Build history of the part. All positions in model axes, mm. A direction names the side the tool comes from. Give positions to 0.01 mm unless a question says otherwise; leave off trailing zeros. Write each loop counter-clockwise with the first axis right and the second up, starting at its lowest first coordinate (ties: lowest second). Pieces come first, ordered by that corner, then holes. Notation, with made-up numbers: (-9.5, -31) -> (44.5, -31) arc R19 ccw to (44.5, 1) -> close; hole circle Ø6 at (-4, 74.25). An arc over 180 degrees is marked (long way). Put each result on its own line as item: value. Start each with the question number.
Item 1: Two-plate mould, pull along X, no slides. Class faces 6 (the cylindrical face through (2.21, -8.26, -1.33)), 7 (the flat face through (0, 0, 1)), 8 (the cylindrical face through (6.31, 10.906, -1.331)): pulls with the +X half, pulls with the -X half, needs draft (parallel to the pull), parting line crosses it, or undercut.
Item 2: Drill centre lines: line 1 along Y through (x, z) = (0, -3.1); line 2 along Y through (x, z) = (-9, -2.3); line 3 along Y through (x, z) = (-9.5, -1.75). Where is each one in solid material? Low to high.
Item 3: Slice it at C-C, the plane y = -10. Give the number of separate pieces and of enclosed holes in the cut face, plus the area to 3 significant figures.
Item 4: Slice it at A-A, the plane x = 0. List the corners of the cut face in (y, z), plus the area to 3 significant figures.
Item 5: Tool access for faces 1 (the cylindrical face through (8.257, -2.219, -1.331)), 2 (the cylindrical face through (-8.26, -2.21, -1.33)), 3 (the cylindrical face through (-2.21, 8.26, -1.33)), 4 (the cylindrical face through (-2.219, -8.257, -1.331)), 5 (the cylindrical face through (0.54, -2.44, -3.1)): list every direction of +Z, -Z, +X, -X, +Y, -Y with a clear straight run to the whole face (end or side of a thin tool).
```python
from build123d import *

# Parameters (mm, degrees)
EXTRUDE_1_DEPTH      = 1
EXTRUDE_1_DEPTH_BACK = 3.597865908
SKETCH_2_R           = 2.5
CUT_EXTRUDE_1_DEPTH  = 1


with BuildPart() as part:
    # 草图1 → 凸台-拉伸1 (new, two sides: drawn at the far end of the back side and taken through both)
    with BuildSketch(Plane.XY.offset(-EXTRUDE_1_DEPTH_BACK)):
        with BuildLine():
            ThreePointArc((-2.640449702, -8.132067718), (-2.212902836, -8.258665815), (-1.779337339, -8.36280208))
            add(Edge.make_bspline(
                [(-0.798942675, -12.574644751), (-1.838065444, -11.330781503), (-1.08287755, -9.669464778), (-1.779337339, -8.36280208)],
                knots=[0, 0, 0, 0, 1, 1, 1, 1], degree=3))
            ThreePointArc((-0.798942675, -12.574644751), (0, -12.6), (0.798942675, -12.574644751))
            add(Edge.make_bspline(
                [(0.798942675, -12.574644751), (1.838065444, -11.330781503), (1.08287755, -9.669464778), (1.779337339, -8.36280208)],
                knots=[0, 0, 0, 0, 1, 1, 1, 1], degree=3))
            ThreePointArc((1.779337339, -8.36280208), (2.212902836, -8.258665815), (2.640449702, -8.132067718))
            add(Edge.make_bspline(
                [(5.595417723, -11.289433135), (4.073579383, -10.731777349), (3.896932922, -8.915440914), (2.640449702, -8.132067718)],
                knots=[0, 0, 0, 0, 1, 1, 1, 1], degree=3))
            ThreePointArc((5.595417723, -11.289433135), (6.3, -10.911920088), (6.979227028, -10.49049046))
            add(Edge.make_bspline(
                [(6.979227028, -10.49049046), (7.25720212, -8.893711904), (5.772531856, -7.832563364), (5.722352378, -6.352730379)],
                knots=[0, 0, 0, 0, 1, 1, 1, 1], degree=3))
            ThreePointArc((5.722352378, -6.352730379), (6.045762979, -6.045762979), (6.352730379, -5.722352378))
            add(Edge.make_bspline(
                [(10.49049046, -6.979227028), (8.893711904, -7.25720212), (7.832563364, -5.772531856), (6.352730379, -5.722352378)],
                knots=[0, 0, 0, 0, 1, 1, 1, 1], degree=3))
            ThreePointArc((10.49049046, -6.979227028), (10.911920088, -6.3), (11.289433135, -5.595417723))
            add(Edge.make_bspline(
                [(11.289433135, -5.595417723), (10.731777349, -4.073579383), (8.915440914, -3.896932922), (8.132067718, -2.640449702)],
                knots=[0, 0, 0, 0, 1, 1, 1, 1], degree=3))
            ThreePointArc((8.132067718, -2.640449702), (8.258665815, -2.212902836), (8.36280208, -1.779337339))
            add(Edge.make_bspline(
                [(12.574644751, -0.798942675), (11.330781503, -1.838065444), (9.669464778, -1.08287755), (8.36280208, -1.779337339)],
                knots=[0, 0, 0, 0, 1, 1, 1, 1], degree=3))
            ThreePointArc((12.574644751, -0.798942675), (12.6, 0), (12.574644751, 0.798942675))
            add(Edge.make_bspline(
                [(12.574644751, 0.798942675), (11.330781503, 1.838065444), (9.669464778, 1.08287755), (8.36280208, 1.779337339)],
                knots=[0, 0, 0, 0, 1, 1, 1, 1], degree=3))
            ThreePointArc((8.36280208, 1.779337339), (8.258665815, 2.212902836), (8.132067718, 2.640449702))
            add(Edge.make_bspline(
                [(11.289433135, 5.595417723), (10.731777349, 4.073579383), (8.915440914, 3.896932922), (8.132067718, 2.640449702)],
                knots=[0, 0, 0, 0, 1, 1, 1, 1], degree=3))
            ThreePointArc((11.289433135, 5.595417723), (10.911920088, 6.3), (10.49049046, 6.979227028))
            add(Edge.make_bspline(
                [(10.49049046, 6.979227028), (8.893711904, 7.25720212), (7.832563364, 5.772531856), (6.352730379, 5.722352378)],
                knots=[0, 0, 0, 0, 1, 1, 1, 1], degree=3))
            ThreePointArc((6.352730379, 5.722352378), (6.045762979, 6.045762979), (5.722352378, 6.352730379))
            add(Edge.make_bspline(
                [(6.979227028, 10.49049046), (7.25720212, 8.893711904), (5.772531856, 7.832563364), (5.722352378, 6.352730379)],
                knots=[0, 0, 0, 0, 1, 1, 1, 1], degree=3))
            ThreePointArc((6.979227028, 10.49049046), (6.3, 10.911920088), (5.595417723, 11.289433135))
            add(Edge.make_bspline(
                [(5.595417723, 11.289433135), (4.073579383, 10.731777349), (3.896932922, 8.915440914), (2.640449702, 8.132067718)],
                knots=[0, 0, 0, 0, 1, 1, 1, 1], degree=3))
            ThreePointArc((2.640449702, 8.132067718), (2.212902836, 8.258665815), (1.779337339, 8.36280208))
            add(Edge.make_bspline(
                [(0.798942675, 12.574644751), (1.838065444, 11.330781503), (1.08287755, 9.669464778), (1.779337339, 8.36280208)],
                knots=[0, 0, 0, 0, 1, 1, 1, 1], degree=3))
            ThreePointArc((0.798942675, 12.574644751), (0, 12.6), (-0.798942675, 12.574644751))
            add(Edge.make_bspline(
                [(-0.798942675, 12.574644751), (-1.838065444, 11.330781503), (-1.08287755, 9.669464778), (-1.779337339, 8.36280208)],
                knots=[0, 0, 0, 0, 1, 1, 1, 1], degree=3))
            ThreePointArc((-1.779337339, 8.36280208), (-2.212902836, 8.258665815), (-2.640449702, 8.132067718))
            add(Edge.make_bspline(
                [(-5.595417723, 11.289433135), (-4.073579383, 10.731777349), (-3.896932922, 8.915440914), (-2.640449702, 8.132067718)],
                knots=[0, 0, 0, 0, 1, 1, 1, 1], degree=3))
            ThreePointArc((-5.595417723, 11.289433135), (-6.3, 10.911920088), (-6.979227028, 10.49049046))
            add(Edge.make_bspline(
                [(-6.979227028, 10.49049046), (-7.25720212, 8.893711904), (-5.772531856, 7.832563364), (-5.722352378, 6.352730379)],
                knots=[0, 0, 0, 0, 1, 1, 1, 1], degree=3))
            ThreePointArc((-5.722352378, 6.352730379), (-6.045762979, 6.045762979), (-6.352730379, 5.722352378))
            add(Edge.make_bspline(
                [(-10.49049046, 6.979227028), (-8.893711904, 7.25720212), (-7.832563364, 5.772531856), (-6.352730379, 5.722352378)],
                knots=[0, 0, 0, 0, 1, 1, 1, 1], degree=3))
            ThreePointArc((-10.49049046, 6.979227028), (-10.911920088, 6.3), (-11.289433135, 5.595417723))
            add(Edge.make_bspline(
                [(-11.289433135, 5.595417723), (-10.731777349, 4.073579383), (-8.915440914, 3.896932922), (-8.132067718, 2.640449702)],
                knots=[0, 0, 0, 0, 1, 1, 1, 1], degree=3))
            ThreePointArc((-8.132067718, 2.640449702), (-8.258665815, 2.212902836), (-8.36280208, 1.779337339))
            add(Edge.make_bspline(
                [(-12.574644751, 0.798942675), (-11.330781503, 1.838065444), (-9.669464778, 1.08287755), (-8.36280208, 1.779337339)],
                knots=[0, 0, 0, 0, 1, 1, 1, 1], degree=3))
            ThreePointArc((-12.574644751, 0.798942675), (-12.6, 0), (-12.574644751, -0.798942675))
            add(Edge.make_bspline(
                [(-12.574644751, -0.798942675), (-11.330781503, -1.838065444), (-9.669464778, -1.08287755), (-8.36280208, -1.779337339)],
                knots=[0, 0, 0, 0, 1, 1, 1, 1], degree=3))
            ThreePointArc((-8.36280208, -1.779337339), (-8.258665815, -2.212902836), (-8.132067718, -2.640449702))
            add(Edge.make_bspline(
                [(-11.289433135, -5.595417723), (-10.731777349, -4.073579383), (-8.915440914, -3.896932922), (-8.132067718, -2.640449702)],
                knots=[0, 0, 0, 0, 1, 1, 1, 1], degree=3))
            ThreePointArc((-11.289433135, -5.595417723), (-10.911920088, -6.3), (-10.49049046, -6.979227028))
            add(Edge.make_bspline(
                [(-10.49049046, -6.979227028), (-8.893711904, -7.25720212), (-7.832563364, -5.772531856), (-6.352730379, -5.722352378)],
                knots=[0, 0, 0, 0, 1, 1, 1, 1], degree=3))
            ThreePointArc((-6.352730379, -5.722352378), (-6.045762979, -6.045762979), (-5.722352378, -6.352730379))
            add(Edge.make_bspline(
                [(-6.979227028, -10.49049046), (-7.25720212, -8.893711904), (-5.772531856, -7.832563364), (-5.722352378, -6.352730379)],
                knots=[0, 0, 0, 0, 1, 1, 1, 1], degree=3))
            ThreePointArc((-6.979227028, -10.49049046), (-6.3, -10.911920088), (-5.595417723, -11.289433135))
            add(Edge.make_bspline(
                [(-5.595417723, -11.289433135), (-4.073579383, -10.731777349), (-3.896932922, -8.915440914), (-2.640449702, -8.132067718)],
                knots=[0, 0, 0, 0, 1, 1, 1, 1], degree=3))
        make_face()
    extrude(amount=EXTRUDE_1_DEPTH + EXTRUDE_1_DEPTH_BACK)

    # 草图2 → 切除-拉伸1 (cut)
    with BuildSketch(Plane(origin=(0, 0, -3.597865908), x_dir=(-1, 0, 0), z_dir=(0, 0, -1))):
        Circle(SKETCH_2_R)
    extrude(amount=-CUT_EXTRUDE_1_DEPTH, mode=Mode.SUBTRACT)


solid = part.part
```
Values follow:
1. face 6: undercut
1. face 7: needs draft
1. face 8: pulls with the +X half
2. line 1: -12.6 to -2.5, 2.5 to 12.6
2. line 2: -6.77 to -3.51, -1.55 to 1.55, 3.51 to 6.77
2. line 3: -6.94 to -3.83, -1.47 to 1.47, 3.83 to 6.94
3. separate pieces: 3
3. enclosed holes: 0
3. area: 39.5 mm2
4. outline: (-12.6, -3.6) -> (-2.5, -3.6) -> (-2.5, -2.6) -> (2.5, -2.6) -> (2.5, -3.6) -> (12.6, -3.6) -> (12.6, 1) -> (-12.6, 1) -> close
4. area: 111 mm2
5. face 1: +Z, -Z, +X
5. face 2: +Z, -Z, -X
5. face 3: +Z, -Z, +Y
5. face 4: +Z, -Z, -Y
5. face 5: -Z
